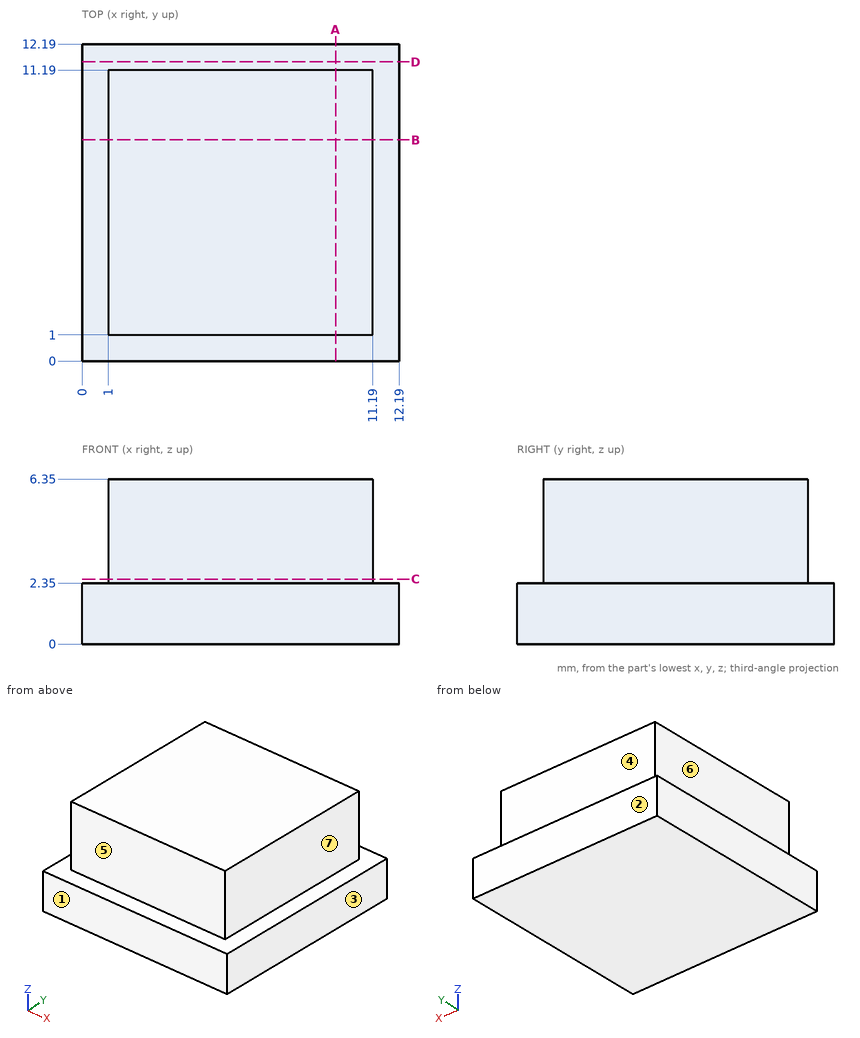
Geometry: see drawing. Coordinates: mm, zero at the bounding-box minimum. A direction names the side the tool comes from. Coordinates: 2 decimals unless noted, no trailing zeros. Write each loop counter-clockwise with the first axis right and the second up, starting at its lowest first coordinate (ties: lowest second). Pieces come first, ordered by that corner, then holes.
1) Pin query (flat end, axial travel): pin 1 Ø1.2 at (x, z) = (8.5, 3.5) entering from -Y; pin 2 Ø1.2 at (x, z) = (7, 4) entering from +Y; pin 3 Ø2 at (y, z) = (6, 4) entering from -X. Return the tip coordinate at first contact, or that it passes through.
2) Section D-D on y = 11.5. Output: boundary loops of the cut face in (x, z).
3) Set-up query: the marked faces 4, 5, 6 and 7. Return all of +Z, -Z, +X, -X, +Y, -Y with unobstructed straight access to the full face (end or side cutting, diameter ignored); none if empty.
4) Section A-A on x = 9.75. Output: boundary loops of the cut face in (y, z), and give its area (3 significant figures).
5) Mould query, pull axis Y, two halves, no side actions, for the marked faces 1, 2 and 3. Classes: pulls with the +Y half, pulls with the -Y half, needs draft (parallel to the pull), parting line crosses it, or undercut.
6) Section C-C on z = 2.5. Output: boundary loops of the cut face in (x, y), and give its area (3 significant figures).
7) Material intervals for line 1 along X through (y, z) = (4.5, 4); line 2 along Z through (x, y) = (0.75, 8), sorted ascending.
Check result:
1. pin 1: stops at y = 1
1. pin 2: stops at y = 11.19
1. pin 3: stops at x = 1
2. outline: (0, 0) - (12.19, 0) - (12.19, 2.35) - (0, 2.35) - close
3. face 4: +Z, +X, -X, +Y
3. face 5: +Z, +X, -X, -Y
3. face 6: +Z, -X, +Y, -Y
3. face 7: +Z, +X, +Y, -Y
4. outline: (0, 0) - (12.19, 0) - (12.19, 2.35) - (11.19, 2.35) - (11.19, 6.35) - (1, 6.35) - (1, 2.35) - (0, 2.35) - close
4. area: 69.4 mm2
5. face 1: pulls with the -Y half
5. face 2: pulls with the +Y half
5. face 3: needs draft
6. outline: (1, 1) - (11.19, 1) - (11.19, 11.19) - (1, 11.19) - close
6. area: 104 mm2
7. line 1: x = 1 to 11.19
7. line 2: z = 0 to 2.35
